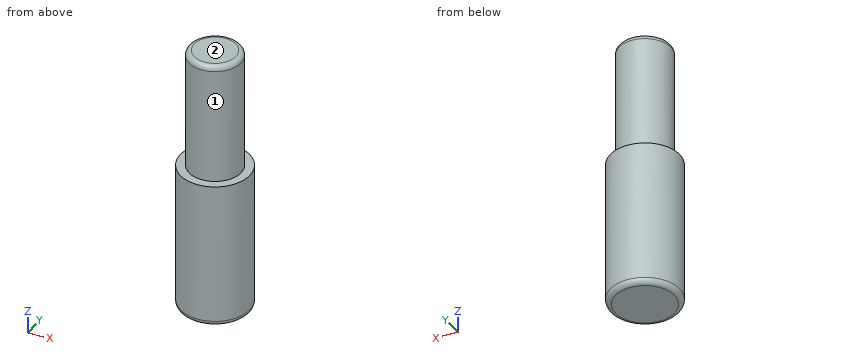
Autodesk Fusion 360 part; units mm, degrees
sketch "Skizze1" plane through (0, 0, 0) normal (0, 0, 1) x (1, 0, 0)
  circle A0 centre (0, 0) radius 2
  dimension "d1" = 4
extrude "Extrusion1" add sketch "Skizze1" along normal blind 8.5
sketch "Skizze2" plane through (0, 0, 8.5) normal (0, 0, 1) x (-1, 0, 0)
  circle A0 centre (0, 0) radius 2
  circle A1 centre (0, 0) radius 1.5
  dimension "d4" = 3
extrude "Extrusion2" add sketch "Skizze2" along normal blind 7 contours A1
fillet "Abrundung1" radius 0.3 1 edges at (1.3985, 0.5424, 15.5)
fillet "Abrundung2" radius 0.3 1 edges at (-1.8647, -0.7232, 0)
The listing builds one solid part. Answer for the finished solid, in the listing's coordinates (mm). Face numbers are marked on the shaded views. A direction names the side the tool comes from. Round coordinates to 2 decimals unless told otherwise and drop trailing zeros. Loops run counter-clockwise (first coordinate to the right, second up) from the corner with the lowest first, then second, coordinate; pieces in that order, holes last. Notation, with made-up numbers: M -3,36 L 23,36 A20 cw 23,45 Z; hole C 14,-13 d5. An arc over 180 degrees is marked long. Return JSON: item names as keys, results as strings.
Q1. Find section D-D, the plane z = 12. Determine the outline of the cut face in (x, y).
Results list:
{"outline": "C 0,0 d3"}
Q2. Find section A-A, the plane y = 0. Determine the outline of the cut face in (x, z).
Results list:
{"outline": "M -2,0.3 A0.3 ccw -1.7,0 L 1.7,0 A0.3 ccw 2,0.3 L 2,8.5 L 1.5,8.5 L 1.5,15.2 A0.3 ccw 1.2,15.5 L -1.2,15.5 A0.3 ccw -1.5,15.2 L -1.5,8.5 L -2,8.5 Z"}
Q3. Find section C-C, the plane z = 2.25. Determine the outline of the cut face in (x, y), plus the area to 3 significant figures.
Results list:
{"outline": "C 0,0 d4", "area": "12.6 mm2"}
Q4. Which of the six approach directions +Z, -Z, +X, -X, +Y, -Y give full straight-line access (tool end or side, diameter ignored) to the marked faces 1 and 2?
Results list:
{"face 1": "+Z", "face 2": "+Z, +X, -X, +Y, -Y"}
Q5. Find the intervals of material crossed by line 1 along X through (y, z) = (-0.1, 2.5); line 2 along Z through (x, y) = (-1.35, 0.75); line 3 along X through (y, z) = (0.05, 8.75), in increasing order. Write a range as from..to.
Results list:
{"line 1": "x = -2..2", "line 2": "z = 0..8.5", "line 3": "x = -1.5..1.5"}
Q6. This flat-tipped pin is pushed along its axis until it touches: pin 1 Ø1 at (x, z) = (-1, 7) entering from -Y. Where does it stop, or does it pass through?
Results list:
{"pin 1": "stops at y = -1.94"}
